```python
from build123d import *

# Parameters (mm, degrees)
SKETCH_1_R          = 4.5
EXTRUDE_1_DEPTH     = 3
SKETCH_2_R          = 2.5
EXTRUDE_2_DEPTH     = 25
EXTRUDE_START       = -25
SKETCH_3_R          = 2
EXTRUDE_3_DEPTH     = 8
CUT_EXTRUDE_START   = 3
CUT_EXTRUDE_1_DEPTH = 2
FILLET_1_R          = 0.5


with BuildPart() as part:
    # 草图1 → 凸台-拉伸1 (new body)
    with BuildSketch(Plane.XY):
        Circle(SKETCH_1_R)
    extrude(amount=EXTRUDE_1_DEPTH)

    # 草图2 → 凸台-拉伸2 (add)
    with BuildSketch(Plane.XY):
        Circle(SKETCH_2_R)
    extrude(amount=-EXTRUDE_2_DEPTH)

    # 草图3 → 凸台-拉伸3 (add)
    with BuildSketch(Plane.XY.offset(EXTRUDE_START)):
        Circle(SKETCH_3_R)
    extrude(amount=-EXTRUDE_3_DEPTH)

    # 草图4 → 切除-拉伸1 (cut)
    with BuildSketch(Plane.XY.offset(CUT_EXTRUDE_START)):
        Polygon((1.732050808, 0), (0.866025404, 1.5), (-0.866025404, 1.5), (-1.732050808, 0), (-0.866025404, -1.5), (0.866025404, -1.5), align=None)
    extrude(amount=-CUT_EXTRUDE_1_DEPTH, mode=Mode.SUBTRACT)

    # 圆角1
    fillet_1_edges = [part.edges().sort_by_distance(p)[0] for p in [
        (-4.5, 0, 3),
    ]]
    fillet(fillet_1_edges, radius=FILLET_1_R)


solid = part.part
```
Input: part model. Units: mm. Frame: model coordinates. A direction names the side the tool comes from. Round coordinates to 2 decimals unless told otherwise and drop trailing zeros. Write each loop counter-clockwise with the first axis right and the second up, starting at its lowest first coordinate (ties: lowest second). Pieces come first, ordered by that corner, then holes. Notation, with made-up numbers: M 46,85.5 L 82,85.5 A25 ccw 82,101.5 Z; hole C 61,0.25 d9. An arc over 180 degrees is marked long. Write each question's results on one line, items separated by ' | '.
Q1. Access query for faces 4 (the face through (0, 0, -33)), 5 (the face through (2, -2, 0)), 6 (the face through (0, 0, 1)). Directions: +Z, -Z, +X, -X, +Y, -Y. A direction counts if a zero-diameter tool reaches every point of the face in a straight line with its end or side. Return the directions, or none.
Results:
face 4: -Z, +X, -X, +Y, -Y | face 5: -Z | face 6: +Z
Q2. Draft query along Y for faces 1 (the face through (-1.305, -0.74, 2.014)), 2 (the face through (-1, 2, -25)), 3 (the face through (0, -2, -29)). Return one class per face: released by +Y, released by -Y, zero draft, split by the parting line, or undercut.
Results:
face 1: undercut | face 2: zero draft | face 3: split by the parting line
Q3. Section query B-B (z = -23.5). Return loops of the section in (x, y).
Results:
outline: C 0,0 d5
Q4. Section query A-A (x = 0). Return loops of the section in (y, z).
Results:
outline: M -4.5,0 L -2.5,0 L -2.5,-25 L -2,-25 L -2,-33 L 2,-33 L 2,-25 L 2.5,-25 L 2.5,0 L 4.5,0 L 4.5,2.5 A0.5 ccw 4,3 L 1.5,3 L 1.5,1 L -1.5,1 L -1.5,3 L -4,3 A0.5 ccw -4.5,2.5 Z
Q5. Pin query (flat end, axial travel): P1, Ø1.5, axis at x = 0.5, y = -0.5, coming from the +Z side; P2, Ø2, axis at x = 1.5, z = -27.5, coming from the -Y side; P3, Ø1, axis at y = 1.5, z = -5, coming from the -X side. Return the tip coordinate at first contact, or that it passes through.
Results:
P1: stops at z = 1 | P2: stops at y = -1.94 | P3: stops at x = -2.29
Q6. Line query: line 1 along Z through (x, y) = (1, -2.5); line 2 along Z through (x, y) = (-1.25, -0.5); line 3 along X through (y, z) = (-1.75, -23.5). Output: solid intervals per line, ascending.
Results:
line 1: z = 0 to 3 | line 2: z = -33 to 1 | line 3: x = -1.79 to 1.79
